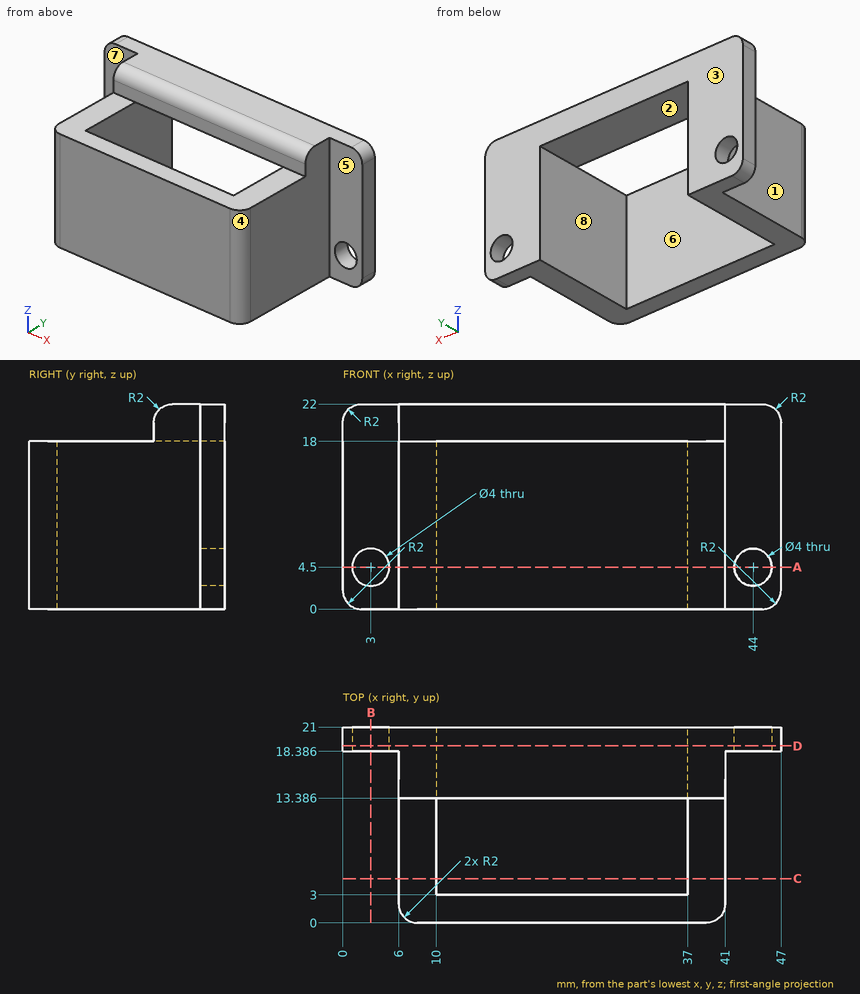
Design review of the part shown in the three views and the two pictorial views. Dimensions are in mm from the part's minimum x, y and z. A direction names the side the tool comes from. Give positions to 0.01 mm unless a question says otherwise; leave off trailing zeros. Loops run counter-clockwise (first coordinate to the right, second up) from the corner with the lowest first, then second, coordinate; pieces in that order, holes last. Notation, with made-up numbers: M 42.5,71 L 89.5,71 A23 ccw 89.5,89 Z; hole C 2,70 d4. An arc over 180 degrees is marked long. Answer as a JSON object with one key per item and string values.
Item 1: We need section A-A (z = 4.5). State the section outline as (x, y) points (1 decimal), and give its area (3 significant figures).
Output values:
{"outline": "M 0,18.4 L 1,18.4 L 1,21 L 0,21 Z; M 5,18.4 L 6,18.4 L 6,2 A2 ccw 8,0 L 39,0 A2 ccw 41,2 L 41,18.4 L 42,18.4 L 42,21 L 37,21 L 37,3 L 10,3 L 10,21 L 5,21 Z; M 46,18.4 L 47,18.4 L 47,21 L 46,21 Z", "area": "258 mm2"}
Item 2: Mouldability with a two-part tool opening along X and no side actions: class the marked faces 1, 2, 3 and 4 as pulls with the +X half, pulls with the -X half, needs draft (parallel to the pull), parting line crosses it, or undercut.
Output values:
{"face 1": "pulls with the -X half", "face 2": "undercut", "face 3": "needs draft", "face 4": "pulls with the +X half"}
Item 3: We need section B-B (x = 3). State the section outline as (y, z) points (1 decimal).
Output values:
{"outline": "M 18.4,0 L 21,0 L 21,2.5 L 18.4,2.5 Z; M 18.4,6.5 L 21,6.5 L 21,22 L 18.4,22 Z"}
Item 4: Wall thickness on line 1 along Z through (x, y) = (3, 20.15); line 2 along X through (y, z) = (15.75, 12.5); line 3 along Y through (x, z) = (27.5, 9.75): over which ranges is each line inside the solid? List them lowest first.
Output values:
{"line 1": "z = 0 to 2.5, 6.5 to 22", "line 2": "x = 6 to 10, 37 to 41", "line 3": "y = 0 to 3"}
Item 5: We need section C-C (y = 4.75). State the section outline as (x, z) points.
Output values:
{"outline": "M 6,0 L 10,0 L 10,18 L 6,18 Z; M 37,0 L 41,0 L 41,18 L 37,18 Z"}
Item 6: Machinability: for the marked faces 5, 6, 7 and 8, which of the approach directions +Z, -Z, +X, -X, +Y, -Y give a long, thin tool a straight path to every point of the face, cutting with its end or side? Answer none if there is none.
Output values:
{"face 5": "+Z, -Z, +X, -Y", "face 6": "+Z, -Z, +Y", "face 7": "+Z, -Z, -X, -Y", "face 8": "-Z, +Y"}
Item 7: We need section D-D (y = 19). State the section outline as (x, z) points.
Output values:
{"outline": "M 0,2 A2 ccw 2,0 L 10,0 L 10,18 L 37,18 L 37,0 L 45,0 A2 ccw 47,2 L 47,20 A2 ccw 45,22 L 2,22 A2 ccw 0,20 Z; hole C 3,4.5 d4; hole C 44,4.5 d4"}
Item 8: For P1, Ø1, axis at x = 32, z = 19, coming from the -Y side; P2, Ø4, axis at x = 20, y = 13, coming from the +Z side; P3, Ø5.5, axis at y = 9.5, z = 11.5, coming from the -X side, all flat-tipped, find the tip position at first contact; note any pin that passes through.
Output values:
{"P1": "stops at y = 13.39", "P2": "stops at z = 21.96", "P3": "stops at x = 6"}
